Check sheet for the modelled part. Datum: model origin and axes. Units: mm. A direction names the side the tool comes from. Round coordinates to 2 decimals unless told otherwise and drop trailing zeros. Order: outer loops, then holes, each group sorted by start corner. A loop starts at its lowest first (then second) coordinate and runs counter-clockwise, first axis right, second up. Notation, with made-up numbers: (48, 6.5) -> (89, 6.5) arc R7 cw to (89, 10.5) -> close; hole circle Ø5 at (23, 45). An arc over 180 degrees is marked (long way). Answer in a Markdown table with one row per item.
from build123d import *

# Parameters (mm, degrees)
CROQUIS2_R              = 15
SALIENTE_EXTRUIR2_DEPTH = 30
CROQUIS3_R              = 11
CORTAR_EXTRUIR1_DEPTH   = 7
CORTAR_EXTRUIR2_START   = -7
CROQUIS4_R              = 11
CORTAR_EXTRUIR2_DEPTH   = 7
CORTAR_EXTRUIR3_REACH   = 33.289
CROQUIS5_R              = 9.5


with BuildPart() as part:
    # Croquis2 → Saliente-Extruir2 (new body)
    with BuildSketch(Plane(origin=(0, 0, 0), x_dir=(1, 0, 0), z_dir=(0, 1, 0))):
        with Locations(Location((0, 0, 0), (0, 0, 270))):
            Circle(CROQUIS2_R)
    extrude(amount=SALIENTE_EXTRUIR2_DEPTH)

    # Croquis3 → Cortar-Extruir1 (cut)
    with BuildSketch(Plane(origin=(0, 30, 0), x_dir=(1, 0, 0), z_dir=(0, 1, 0))):
        with Locations(Location((0, 0, 0), (0, 0, 270))):
            Circle(CROQUIS3_R)
    extrude(amount=-CORTAR_EXTRUIR1_DEPTH, mode=Mode.SUBTRACT)

    # Croquis4 → Cortar-Extruir2 (cut)
    with BuildSketch(Plane(origin=(0, 0, 0), x_dir=(-1, 0, 0), z_dir=(0, -1, 0)).offset(CORTAR_EXTRUIR2_START)):
        with Locations(Location((0, 0, 0), (0, 0, 270))):
            Circle(CROQUIS4_R)
    extrude(amount=CORTAR_EXTRUIR2_DEPTH, mode=Mode.SUBTRACT)

    # Croquis5 → Cortar-Extruir3 (cut, up to next)
    with BuildSketch(Plane(origin=(0, 23, 0), x_dir=(1, 0, 0), z_dir=(0, 1, 0)), mode=Mode.PRIVATE) as cortar_extruir3_sk1:
        with Locations(Location((0, 0, 0), (0, 0, 270))):
            Circle(CROQUIS5_R)
    cortar_extruir3_tool1 = extrude(cortar_extruir3_sk1.sketch, amount=-CORTAR_EXTRUIR3_REACH, mode=Mode.PRIVATE) & part.part
    add(cortar_extruir3_tool1.solids().sort_by_distance((0, 23, 0))[0], mode=Mode.SUBTRACT)


solid = part.part
Item 1: Cross-section at D-D (x = -12.5). Record the boundary of the cut face in (y, z), and give its area (3 significant figures).
Result sheet:
| item | result |
|---|---|
| outline | (0, -8.29) -> (30, -8.29) -> (30, 8.29) -> (0, 8.29) -> close |
| area | 497 mm^2 |
Item 2: Set-up check for faces 1 (the flat face through (0, 23, -10)), 2 (the cylindrical face through (10.74, 3.55, -2.38)), 3 (the cylindrical face through (-5.78, 15.11, -7.54)): record each of +Z, -Z, +X, -X, +Y, -Y from which the full face is reachable in a straight line by a thin tool's end or side.
Result sheet:
| item | result |
|---|---|
| face 1 | +Y |
| face 2 | -Y |
| face 3 | +Y, -Y |
Item 3: Scan lines: line 1 (X direction, y = 4.5, z = 0); line 2 (Z direction, x = 1.5, y = 13.5); line 3 (X direction, y = 18, z = 0). Record each from-to range of solid material in increasing order. Write a range as [from, to].
Result sheet:
| item | result |
|---|---|
| line 1 | x = [-15, -11], [11, 15] |
| line 2 | z = [-14.92, -9.38], [9.38, 14.92] |
| line 3 | x = [-15, -9.5], [9.5, 15] |
Item 4: Mould release check, pull along X, two halves, no side actions. Record for faces 4 (the flat face through (0, 7, -10)), 5 (the cylindrical face through (-10.74, 26.55, -2.38)), 6 (the cylindrical face through (0.66, 14.79, -14.985)), 7 (the flat face through (10, 0, -5)): pulls with the +X half, pulls with the -X half, needs draft (parallel to the pull), parting line crosses it, or undercut.
Result sheet:
| item | result |
|---|---|
| face 4 | undercut |
| face 5 | undercut |
| face 6 | parting line crosses it |
| face 7 | needs draft |
Item 5: Cross-section at A-A (x = 0). Record the boundary of the cut face in (y, z), and give its area (3 significant figures).
Result sheet:
| item | result |
|---|---|
| outline | (0, -15) -> (30, -15) -> (30, -11) -> (23, -11) -> (23, -9.5) -> (7, -9.5) -> (7, -11) -> (0, -11) -> close; (0, 11) -> (7, 11) -> (7, 9.5) -> (23, 9.5) -> (23, 11) -> (30, 11) -> (30, 15) -> (0, 15) -> close |
| area | 288 mm^2 |
Item 6: Cross-section at B-B (z = 0). Record the boundary of the cut face in (x, y), and give its area (3 significant figures).
Result sheet:
| item | result |
|---|---|
| outline | (-15, 0) -> (-11, 0) -> (-11, 7) -> (-9.5, 7) -> (-9.5, 23) -> (-11, 23) -> (-11, 30) -> (-15, 30) -> close; (9.5, 7) -> (11, 7) -> (11, 0) -> (15, 0) -> (15, 30) -> (11, 30) -> (11, 23) -> (9.5, 23) -> close |
| area | 288 mm^2 |
Item 7: Depth check by flat-ended pin: P1, Ø13, axis at x = 0, z = 0, coming from the -Y side; P2, Ø4, axis at y = 11, z = -9, coming from the -X side; P3, Ø4, axis at x = 9.5, y = 26.5, coming from the +Z side; P4, Ø4, axis at x = 10.5, y = 14.5, coming from the -Z side. Enter the tip coordinate at first touch or a pass-through.
Result sheet:
| item | result |
|---|---|
| P1 | passes through |
| P2 | stops at x = -13.27 |
| P3 | stops at z = 12.99 |
| P4 | stops at z = -12.36 |
Item 8: Cross-section at C-C (y = 19.75). Record the boundary of the cut face in (x, z).
Result sheet:
| item | result |
|---|---|
| outline | circle Ø30 at (0, 0); hole circle Ø19 at (0, 0) |
